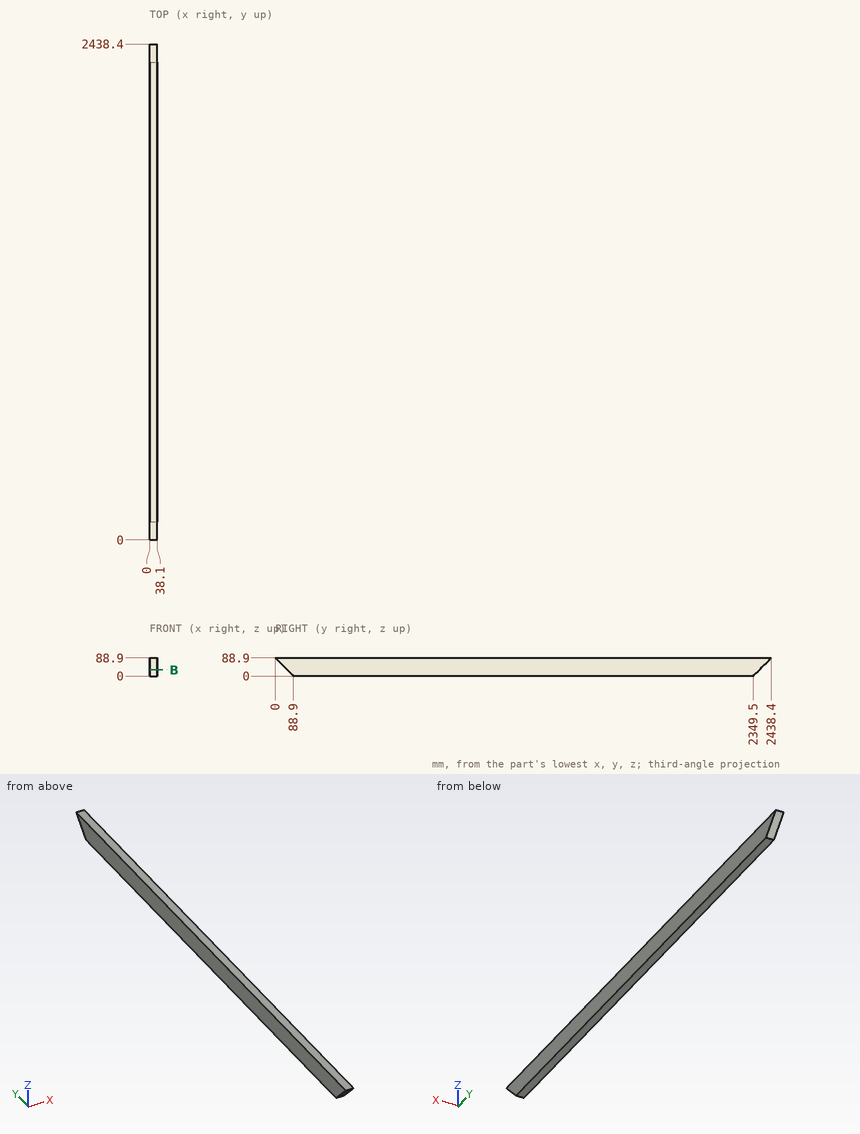
Answer from the drawing. Dimensions are ordinates in mm from the lowest x, y and z of the part. Round coordinates to 2 decimals unless told otherwise and drop trailing zeros. Loops run counter-clockwise (first coordinate to the right, second up) from the corner with the lowest first, then second, coordinate; pieces in that order, holes last.
(1) Each of these flat-tipped pins is pushed along its axis until it touches: P1, Ø1, axis at x = 23.5, z = 71, coming from the +Y side; P2, Ø2, axis at x = 28, z = 57.5, coming from the +Y side; P3, Ø1.5, axis at x = 7.5, z = 26.5, coming from the +Y side. Where does it stop, or does it pass through?
Computed values:
P1: stops at y = 2421
P2: stops at y = 2408
P3: stops at y = 2376.75
(2) The part is cut by section B-B, the plane z = 30. Give the vertices of the cut face in (x, y).
Computed values:
outline: (0, 58.9) - (38.1, 58.9) - (38.1, 2379.5) - (0, 2379.5) - close
(3) Find the intervals of material crossed by L1, parallel to Y at x = 33, z = 53; L2, parallel to Y at x = 21.5, z = 22.5, in increasing order.
Computed values:
L1: y = 35.9 to 2402.5
L2: y = 66.4 to 2372
